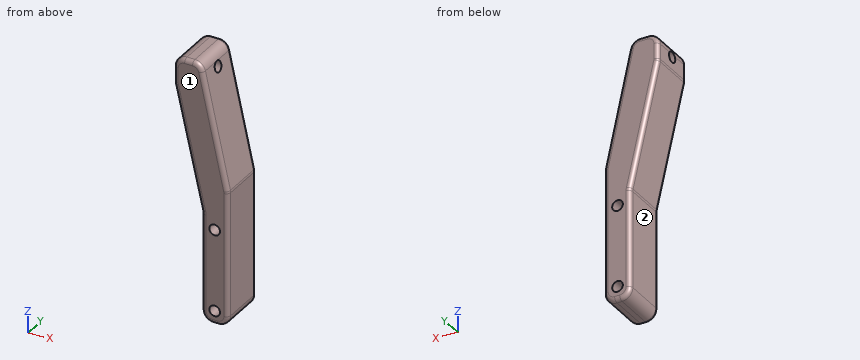
from build123d import *

# Parameters (mm, degrees)
SKETCH2_R           = 2.5
BOSS_EXTRUDE1_DEPTH = 22.2504
CUT_EXTRUDE1_REACH  = 127.286
SKETCH3_R           = 2.5
FILLET2_R           = 5
FILLET3_R           = 2


with BuildPart() as part:
    # Sketch2 → Boss-Extrude1 (new body)
    with BuildSketch(Plane(origin=(0, 0, 0), x_dir=(1, 0, 0), z_dir=(0, 1, 0))):
        Polygon((-25.4, -107.95), (-12.35, -50.8), (-12.35, 0), (0, 0), (0, -63.5), (-12.7, -120.65), (-25.4, -120.65), align=None)
        with Locations(Location((-6.35, -44.45, 0), (0, 0, 90))):
            Circle(SKETCH2_R, mode=Mode.SUBTRACT)
        with Locations(Location((-6.35, -6.35, 0), (0, 0, 90))):
            Circle(SKETCH2_R, mode=Mode.SUBTRACT)
    extrude(amount=BOSS_EXTRUDE1_DEPTH)

    # Cut-Extrude1: up to this plane
    cut_extrude1_end = Plane(origin=(13.447058824, 22.2504, 2.988235294), z_dir=(-0.9761870601839527, 0, -0.21693045781865627))
    # Sketch3 → Cut-Extrude1 (cut, up to the surface)
    with BuildSketch(Plane.ZY.offset(25.4), mode=Mode.PRIVATE) as cut_extrude1_sk1:
        with Locations((114.3, 11.1252)):
            Circle(SKETCH3_R)
    cut_extrude1_tool1 = split(extrude(cut_extrude1_sk1.sketch, amount=-CUT_EXTRUDE1_REACH, mode=Mode.PRIVATE), bisect_by=cut_extrude1_end, keep=Keep.BOTH, mode=Mode.PRIVATE)
    add(cut_extrude1_tool1.solids().sort_by_distance((-25.4, 11.1252, 114.3))[0], mode=Mode.SUBTRACT)

    # Fillet2
    # the kernel refuses this fillet: 5 mm, written as the material it adds along each edge
    with BuildSketch(Plane(origin=(-12.35, 0, 50.8), x_dir=(-0.22261635970063726, 0, 0.9749061269648666), z_dir=(0, 1, 0))) as fillet2_piece_1:
        with BuildLine():
            CenterArc((FILLET2_R * 0.112722501926, -FILLET2_R), FILLET2_R, 90, 12.862751019)
            Line((-FILLET2_R * 0.109893857775, -FILLET2_R * 0.0250938730351), (0, 0))
            Line((0, 0), (FILLET2_R * 0.112722501926, 0))
        make_face()
    extrude(amount=22.2504)
    # the kernel refuses this fillet: 5 mm, written as the material it takes off along each edge
    with BuildSketch(Plane(origin=(-12.35, -12.5, 0), x_dir=(0, 0, 1), z_dir=(0, 1, 0)), Plane(origin=(0, -12.5, 0), x_dir=(-1, 0, 0), z_dir=(0, 1, 0))) as fillet2_2_piece_1:
        with BuildLine():
            CenterArc((FILLET2_R, FILLET2_R), FILLET2_R, 180, 90)
            Line((0, FILLET2_R), (0, 0))
            Line((0, 0), (FILLET2_R, 0))
        make_face()
    extrude(amount=47.2504, mode=Mode.SUBTRACT)
    with BuildSketch(Plane(origin=(0, -1.372152858, 63.5), x_dir=(0, 0, -1), z_dir=(0, 1, 0))) as fillet2_2_piece_2:
        with BuildLine():
            CenterArc((FILLET2_R * 0.109772228646, FILLET2_R), FILLET2_R, 257.471192291, 12.528807709)
            Line((-FILLET2_R * 0.107158229172, FILLET2_R * 0.023812939816), (0, 0))
            Line((0, 0), (FILLET2_R * 0.109772228646, 0))
        make_face()
    extrude(amount=24.994705716, mode=Mode.SUBTRACT)
    with BuildSketch(Plane(origin=(-12.7, -10.02714508, 120.65), x_dir=(0.21693045781865597, 0, -0.9761870601839527), z_dir=(0, 1, 0))) as fillet2_2_piece_3:
        with BuildLine():
            CenterArc((FILLET2_R * 0.802171606366, FILLET2_R), FILLET2_R, 192.528807709, 77.471192291)
            Line((-FILLET2_R * 0.174015453818, FILLET2_R * 0.783069542181), (0, 0))
            Line((0, 0), (FILLET2_R * 0.802171606366, 0))
        make_face()
    extrude(amount=42.304690159, mode=Mode.SUBTRACT)
    with BuildSketch(Plane(origin=(-25.4, -12.5, 120.65), x_dir=(0, 0, -1), z_dir=(0, 1, 0))) as fillet2_2_piece_4:
        with BuildLine():
            CenterArc((FILLET2_R, -FILLET2_R), FILLET2_R, 90, 90)
            Line((0, -FILLET2_R), (0, 0))
            Line((0, 0), (FILLET2_R, 0))
        make_face()
    extrude(amount=47.2504, mode=Mode.SUBTRACT)
    with BuildSketch(Plane(origin=(-25.4, -1.409031274, 107.95), x_dir=(0.2226163597006375, 0, -0.9749061269648664), z_dir=(0, 1, 0))) as fillet2_2_piece_5:
        with BuildLine():
            CenterArc((FILLET2_R * 0.112722501926, -FILLET2_R), FILLET2_R, 90, 12.862751019)
            Line((-FILLET2_R * 0.109893857775, -FILLET2_R * 0.0250938730351), (0, 0))
            Line((0, 0), (FILLET2_R * 0.112722501926, 0))
        make_face()
    extrude(amount=25.068462548, mode=Mode.SUBTRACT)

    # Fillet3
    fillet3_edges = [part.edges().sort_by_distance(p)[0] for p in [
        (-6.175, 0, 0),
        (-6.175, 22.2504, 0),
        (-18.875, 0, 79.375),
        (-12.35, 0, 27.618193745),
        (0, 0, 33.975569428),
        (-5.974493715, 0, 90.385221717),
        (-18.555429016, 0, 120.65),
        (-25.4, 0, 112.081806255),
        (-13.582221064, 0, 119.550209061),
        (-23.935533906, 0, 119.185533906),
        (-25.368533646, 0, 107.953546966),
        (-10.885533906, 0, 1.464466094),
        (-0.029855309, 0, 63.496722716),
        (-1.464466094, 0, 1.464466094),
        (0, 22.2504, 33.975569428),
        (-18.875, 22.2504, 79.375),
        (-25.4, 22.2504, 112.081806255),
        (-18.555429016, 22.2504, 120.65),
        (-5.974493715, 22.2504, 90.385221717),
        (-12.35, 22.2504, 27.618193745),
        (-13.582221064, 22.2504, 119.550209061),
        (-23.935533906, 22.2504, 119.185533906),
        (-25.368533646, 22.2504, 107.953546966),
        (-10.885533906, 22.2504, 1.464466094),
        (-0.029855309, 22.2504, 63.496722716),
        (-1.464466094, 22.2504, 1.464466094),
        (-12.381466354, 0, 50.796453034),
        (-12.381466354, 22.2504, 50.796453034),
    ]]
    fillet(fillet3_edges, radius=FILLET3_R)


solid = part.part
The listing builds one solid part. Answer for the finished solid, in the listing's coordinates (mm). Face numbers are marked on the shaded views. A direction names the side the tool comes from. Round coordinates to 2 decimals unless told otherwise and drop trailing zeros. Write each loop counter-clockwise with the first axis right and the second up, starting at its lowest first coordinate (ties: lowest second). Pieces come first, ordered by that corner, then holes. Notation, with made-up numbers: (-31.75, 67.25) - (9.25, 67.25) arc R21 ccw to (9.25, 77.25) - close; hole circle Ø2 at (48, -33). An arc over 180 degrees is marked (long way). Use a Markdown table: item, result. Add a question column.
1. The part is cut by section C-C (z = 43). Write down the section's boundary in (x, y).
2. The part is cut by section B-B (z = 6.35). Write down the section's boundary in (x, y), and give its area (3 significant figures).
3. Flat-ended cylindrical pins translate along their axes: P1, Ø1.5, axis at y = 17.5, z = 39.5, coming from the -X side; P2, Ø4, axis at x = -2.5, y = 12.5, coming from the -Z side; P3, Ø4, axis at x = -6.35, z = 44.45, coming from the -Y side; P4, Ø2, axis at y = 11.5, z = 73.5, coming from the +X side. Find the tip coordinate at first contact, or state that the pin passes through.
4. The part is cut by section A-A (y = 4.75). Write down the section's boundary in (x, z).
5. Consider line 1 (Y direction, x = -14.75, z = 114.3); line 2 (X direction, y = 13, z = 44.45); line 3 (X direction, y = 10.5, z = 21). Determine where each line is inside the solid, lowest interval first.
6. A tool of negligible diameter and unlimited length cuts with its end or side. For the marked faces 1 and 2, from which of +Z, -Z, +X, -X, +Y, -Y can it reach the whole face along a straight path? Write none if from no direction.
Reported:
| question | item | result |
|---|---|---|
| 1 | outline | (-12.35, 2) arc R2 ccw to (-10.35, 0) - (-8.39, 0) - (-8.39, 22.25) - (-10.35, 22.25) arc R2 ccw to (-12.35, 20.25) - close; (-4.31, 0) - (-2, 0) arc R2 ccw to (0, 2) - (0, 20.25) arc R2 ccw to (-2, 22.25) - (-4.31, 22.25) - close |
| 2 | outline | (-12.35, 2) arc R2 ccw to (-10.35, 0) - (-8.85, 0) - (-8.85, 22.25) - (-10.35, 22.25) arc R2 ccw to (-12.35, 20.25) - close; (-3.85, 0) - (-2, 0) arc R2 ccw to (0, 2) - (0, 20.25) arc R2 ccw to (-2, 22.25) - (-3.85, 22.25) - close |
| 2 | area | 160 mm^2 |
| 3 | P1 | x = -12.35 |
| 3 | P2 | z = 0.03 |
| 3 | P3 | through |
| 3 | P4 | x = -2 |
| 4 | outline | (-25.4, 108.51) arc R5 ccw to (-25.27, 107.4) - (-12.48, 51.35) arc R5 cw to (-12.35, 50.24) - (-12.35, 5) arc R5 ccw to (-7.35, 0) - (-5, 0) arc R5 ccw to (0, 5) - (0, 62.95) arc R5 ccw to (-0.12, 64.04) - (-11.83, 116.73) arc R5 ccw to (-16.71, 120.65) - (-20.4, 120.65) arc R5 ccw to (-25.4, 115.65) - close; hole circle Ø5 at (-6.35, 6.35); hole circle Ø5 at (-6.35, 44.45) |
| 5 | line 1 | 0 to 8.63, 13.63 to 22.25 |
| 5 | line 2 | -12.35 to -8.85, -3.85 to 0 |
| 5 | line 3 | -12.35 to 0 |
| 6 | face 1 | +Z, -Z, +X, -X, -Y |
| 6 | face 2 | -Z, -X, +Y, -Y |
